```python
from build123d import *

# Parameters (mm, degrees)
BOSS_EXTRU_1_DEPTH         = 58
ESQUISSE2_R                = 4
ESQUISSE2_R_2              = 9
ENL_V_MAT_EXTRU_1_DEPTH    = 140.874944147
ESQUISSE3_R                = 11
ENL_V_MAT_EXTRU_2_DEPTH    = 3.5
R_P_TITION_LIN_AIRE1_COUNT = 2
R_P_TITION_LIN_AIRE1_PITCH = 40
TROU_TARAUD_M101_D         = 8.5


with BuildPart() as part:
    # Esquisse1 → Boss.-Extru.1 (new body)
    with BuildSketch(Plane(origin=(0, 0, 0), x_dir=(0, 0, -1), z_dir=(1, 0, 0))):
        Polygon((0, 0), (0, 10), (6, 10), (6, 50), (0, 50), (0, 108), (3, 108), (3, 125), (14, 125), (24, 115), (24, 110), (19, 110), (19, 8), (11, 0), align=None)
    extrude(amount=BOSS_EXTRU_1_DEPTH)

    # Esquisse2 → Enlèv. mat.-Extru.1 (cut, through all)
    with BuildSketch(Plane.XY):
        with Locations((49, 90.5)):
            Circle(ESQUISSE2_R)
        with Locations((9, 90.5)):
            Circle(ESQUISSE2_R)
        with Locations((29, 90.5)):
            Circle(ESQUISSE2_R_2)
        with BuildLine():
            Line((58, 0), (43, 0))
            Line((43, 0), (43, 66))
            ThreePointArc((43, 66), (44.464466094, 69.535533906), (48, 71))
            Line((48, 71), (58, 71))
            Line((58, 71), (58, 0))
        make_face()
        with BuildLine():
            Line((15, 0), (15, 66))
            ThreePointArc((15, 66), (13.535533906, 69.535533906), (10, 71))
            Line((10, 71), (0, 71))
            Line((0, 71), (0, 0))
            Line((0, 0), (15, 0))
        make_face()
    extrude(amount=-ENL_V_MAT_EXTRU_1_DEPTH, mode=Mode.SUBTRACT)

    # Esquisse3 → Enlèv. mat.-Extru.2 (cut)
    with BuildSketch(Plane(origin=(0, 0, -19), x_dir=(-1, 0, 0), z_dir=(0, 0, -1))):
        with Locations(Location((-29, 90.5, 0), (0, 0, 90))):
            Circle(ESQUISSE3_R)
    extrude(amount=-ENL_V_MAT_EXTRU_2_DEPTH, mode=Mode.SUBTRACT)

    # Esquisse5 → Trou taraudé M61 (revolve, cut)
    with BuildSketch(Plane(origin=(49, 117, -3), x_dir=(0, -1, 0), z_dir=(1, 0, 0))):
        Polygon((0, 0), (0, 16.502151548), (2.5, 15), (2.5, 0.866025404), (4, 0), align=None)
    trou_taraud_m61 = revolve(axis=Axis((49, 117, 3.35), (0, 0, -1)), mode=Mode.SUBTRACT)

    # Répétition linéaire1: Trou taraudé M61 ×2
    with Locations(*[(-i * R_P_TITION_LIN_AIRE1_PITCH, 0, 0) for i in range(1, R_P_TITION_LIN_AIRE1_COUNT)]):
        add(trou_taraud_m61, mode=Mode.SUBTRACT)

    # Trou taraudé M101 (through all)
    with Locations(Plane.XY.offset(-6)):
        with Locations((29, 30)):
            Hole(TROU_TARAUD_M101_D / 2)


solid = part.part
```
Geometry check sheet. Reference: the model listing, model coordinates, mm. A direction names the side the tool comes from. Coordinates: 2 decimals unless noted, no trailing zeros. Write each loop counter-clockwise with the first axis right and the second up, starting at its lowest first coordinate (ties: lowest second). Pieces come first, ordered by that corner, then holes. Notation, with made-up numbers: (86.25, 52.25) -> (138.25, 52.25) arc R8 cw to (138.25, 60.25) -> close; hole circle Ø2 at (-18.5, 60.25). An arc over 180 degrees is marked (long way). Use CSV: the item, a comma, the result in double quotes. Start each with the question number.
Item 1: Cross-section at D-D, the plane z = -22. Record the cut outline in (x, y).
Item 2: Cross-section at B-B, the plane x = 29. Record the cut outline in (y, z).
Item 3: Depth check by flat-ended pin: pin 1 Ø2 at (x, y) = (12, 74) entering from +Z; pin 2 Ø2.5 at (x, z) = (32, -22) entering from -Y; pin 3 Ø3 at (x, z) = (3.5, -13.5) entering from -Y; pin 4 Ø4 at (y, z) = (29, -8) entering from -X. Enter the tip coordinate at first touch or a pass-through.
Item 4: Mould release check, pull along X, two halves, no side actions. Record for faces 1 (the flat face through (29, 81, -15.5)), 2 (the flat face through (29, 5, 0)), 3 (the flat face through (43, 33, -11)), 4 (the conical face through (48.87, 116.586, -19.241)): released by +X, released by -X, zero draft, split by the parting line, or undercut.
Item 5: Set-up check for faces 5 (the flat face through (29, 50, -3)), 6 (the flat face through (5, 71, -9)), 7 (the flat face through (53, 71, -9)): record each of +Z, -Z, +X, -X, +Y, -Y from which the full face is reachable in a straight line by a thin tool's end or side.
Item 6: Thickness scan on line 1 (X direction, y = 117, z = -14.5); line 2 (Y direction, x = 49, z = -11.75); line 3 (Y direction, x = 8.5, z = -17.25). Record the ranges inside material, lowest first.
Item 7: Cross-section at C-C, the plane y = 30. Record the cut outline in (x, z), plus the area to 4 significant figures.
Item 8: Cross-section at A-A, the plane y = 90.5. Record the cut outline in (x, z).
Answers:
1,outline,"(0, 110) -> (58, 110) -> (58, 117) -> (0, 117) -> close"
2,outline,"(0, -11) -> (8, -19) -> (25.75, -19) -> (25.75, -6) -> (10, -6) -> (10, 0) -> (0, 0) -> close; (34.25, -19) -> (79.5, -19) -> (79.5, -15.5) -> (81.5, -15.5) -> (81.5, 0) -> (50, 0) -> (50, -6) -> (34.25, -6) -> close; (99.5, -15.5) -> (101.5, -15.5) -> (101.5, -19) -> (110, -19) -> (110, -24) -> (115, -24) -> (125, -14) -> (125, -3) -> (108, -3) -> (108, 0) -> (99.5, 0) -> close"
3,pin 1,"z = 0"
3,pin 2,"y = 110"
3,pin 3,"y = 71"
3,pin 4,"x = 15"
4,face 1,"undercut"
4,face 2,"zero draft"
4,face 3,"released by +X"
4,face 4,"undercut"
5,face 5,"+Z, +X, -X"
5,face 6,"+Z, -Z, -X, -Y"
5,face 7,"+Z, -Z, +X, -Y"
6,line 1,"0 to 6.5, 11.5 to 46.5, 51.5 to 58"
6,line 2,"71 to 86.5, 94.5 to 114.5, 119.5 to 125"
6,line 3,"71 to 86.53, 94.47 to 114.55, 119.45 to 121.75"
7,outline,"(15, -19) -> (24.75, -19) -> (24.75, -6) -> (15, -6) -> close; (33.25, -19) -> (43, -19) -> (43, -6) -> (33.25, -6) -> close"
7,area,"253.5 mm^2"
8,outline,"(0, -19) -> (5, -19) -> (5, 0) -> (0, 0) -> close; (13, -19) -> (18, -19) -> (18, -15.5) -> (20, -15.5) -> (20, 0) -> (13, 0) -> close; (38, -15.5) -> (40, -15.5) -> (40, -19) -> (45, -19) -> (45, 0) -> (38, 0) -> close; (53, -19) -> (58, -19) -> (58, 0) -> (53, 0) -> close"
